Answer from the drawing. Dimensions are ordinates in mm from the lowest x, y and z of the part. Coordinates: 2 decimals unless noted, no trailing zeros. Order: outer loops, then holes, each group sorted by start corner. A loop starts at its lowest first (then second) coordinate and runs counter-clockwise, first axis right, second up. Notation, with made-up numbers: (60, 0) - (92, 0) arc R15 cw to (92, 19) - close; hole circle Ø9 at (20, -32). An arc over 180 degrees is marked (long way). Use a Markdown table: item, result. Add a question column.
Item 1: Find the intervals of material crossed by line 1 along X through (y, z) = (30.5, 8.25); line 2 along Y through (x, z) = (8, 0.25), in increasing order.
Item 2: The part is cut by section C-C, the plane y = 4.5. Give the vertices of the cut face in (x, z).
Item 3: The part is cut by section A-A, the plane z = 8. Give the vertices of the cut face in (x, y), then the cut area to 3 significant figures.
Item 4: Flat-ended cylindrical pins translate along their axes: P1, Ø9, axis at x = 8, z = 8, coming from the +Y side; P2, Ø2, axis at x = 11, y = 23.5, coming from the +Z side; P3, Ø4, axis at y = 35, z = 3, coming from the -X side; P4, Ø3, axis at x = 12.5, y = 18.5, coming from the +Z side. Find the tip coordinate at first contact, or state that the pin passes through.
Item 5: The mould has two halves that part along Z. Classify the marked faces 1 and 2: released by +Z, released by -Z, zero draft, split by the parting line, or undercut.
Item 6: The part is cut by section B-B, the plane x = 8. Give the vertices of the cut face in (y, z), then the cut area to 3 significant figures.
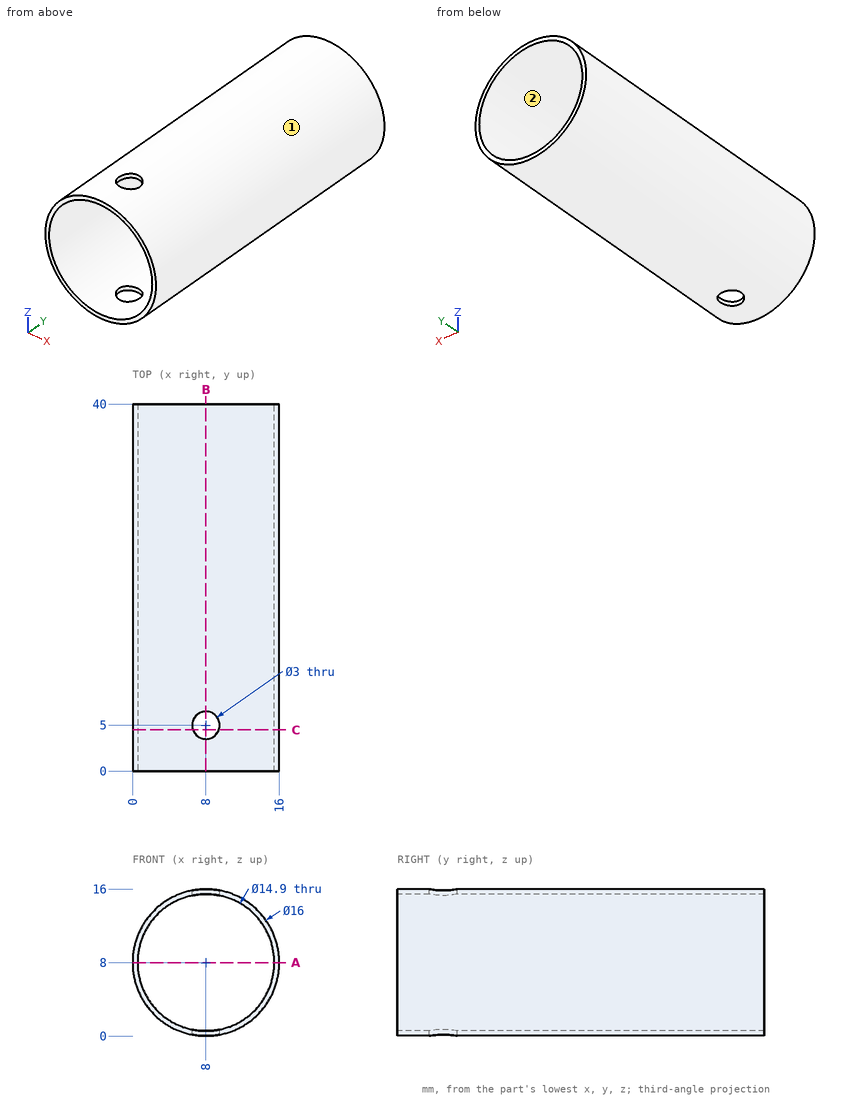
Solution:
| question | item | result |
|---|---|---|
| 1 | line 1 | x = 0 to 0.55, 15.45 to 16 |
| 1 | line 2 | y = 0 to 3.5, 6.5 to 40 |
| 2 | outline | (6.59, 0.13) - (6.59, 0.69) arc R7.45 cw to (6.59, 15.31) - (6.59, 15.87) arc R8 ccw to start; (9.41, 0.13) arc R8 ccw to (9.41, 15.87) - (9.41, 15.31) arc R7.45 cw to (9.41, 0.69) - close |
| 3 | outline | (0, 0) - (0.55, 0) - (0.55, 40) - (0, 40) - close; (15.45, 0) - (16, 0) - (16, 40) - (15.45, 40) - close |
| 3 | area | 44.0 mm2 |
| 4 | P1 | passes through |
| 4 | P2 | stops at z = 15.75 |
| 4 | P3 | stops at x = 0.58 |
| 4 | P4 | stops at z = 15.42 |
| 5 | face 1 | split by the parting line |
| 5 | face 2 | undercut |
| 6 | outline | (0, 0) - (3.5, 0) - (3.5, 0.55) - (0, 0.55) - close; (0, 15.45) - (3.5, 15.45) - (3.5, 16) - (0, 16) - close; (6.5, 0) - (40, 0) - (40, 0.55) - (6.5, 0.55) - close; (6.5, 15.45) - (40, 15.45) - (40, 16) - (6.5, 16) - close |
| 6 | area | 40.7 mm2 |
